Verification items for the finished model (mm, model axes). A direction names the side the tool comes from. Round coordinates to 2 decimals unless told otherwise and drop trailing zeros. Write each loop counter-clockwise with the first axis right and the second up, starting at its lowest first coordinate (ties: lowest second). Pieces come first, ordered by that corner, then holes. Notation, with made-up numbers: M -22.75,49.5 L -0.75,49.5 A16 ccw -0.75,75.5 Z; hole C 54.5,-25 d8. An arc over 180 degrees is marked long. One line per item, written item: value. Start each with the question number.
Item 1: Section check D-D, the plane y = 36. Record the cut outline in (x, z).
Item 2: Thickness scan on probe 1 along X at (y, z) = (-29, 0) (3 decimals); probe 2 along X at (y, z) = (-10.5, 0); probe 3 along X at (y, z) = (26, 0). Record the ranges inside material, lowest first. Write a range as from..to.
Item 3: Gauge pin test, flat ends, axial feed: pin 1 (6 mm diameter, centred on x = 32.5, z = -32, fed in from -Y); pin 2 (6 mm diameter, centred on y = 33.5, z = -19, fed in from -X); pin 3 (3 mm diameter, centred on x = -40, y = -30, fed in from +Z); pin 4 (8 mm diameter, centred on x = 10.5, y = 30.5, fed in from +Z). Record the tip position at first contact, or that the pin passes through.
Item 4: Section check A-A, the plane y = -16.5. Record the cut outline in (x, z) (3 decimals), then the cut area to 3 significant figures.
Item 5: Draft check along X on faces 1 (the face through (18, -30.48, 17)), 2 (the face through (-10.4, 15.24, 10.4)), 3 (the face through (46.492, -23.97, -10.324)). Enter one of: +X half, -X half, draft (parallel to the pull), parting line (faces both ways), or undercut.
Item 6: Tool access check on faces 4 (the face through (-30.911, -6.261, -40.313)), 5 (the face through (0, 20.574, 0)), 6 (the face through (0, 5.08, 0)). Record the directions out of +Z, -Z, +X, -X, +Y, -Y that give a thin tool (end or side, any length) a straight path to the whole face; none if there is none.
from build123d import *

# Parameters (mm, degrees)
SKETCH1_R                = 50.8
SKETCH1_R_2              = 39.116
BOSS_EXTRUDE1_DEPTH      = 12.7
BOSS_EXTRUDE2_DEPTH      = 20.32
BOSS_EXTRUDE2_DEPTH_BACK = 2.54
SKETCH2_R                = 47.625
SKETCH2_R_2              = 39.116
BOSS_EXTRUDE3_DEPTH      = 7.62
BOSS_EXTRUDE3_DEPTH_BACK = 5.08
SKETCH4_R                = 41.91
BOSS_EXTRUDE4_START      = -2.54
SKETCH5_R                = 24.13
BOSS_EXTRUDE4_DEPTH      = 45.72
BOSS_EXTRUDE5_START      = -2.54
SKETCH6_R                = 14.224
BOSS_EXTRUDE5_DEPTH      = 29.21
SKETCH7_R                = 16.51
CUT_EXTRUDE1_DEPTH       = 50.8
SKETCH8_R                = 5.08
CUT_EXTRUDE2_DEPTH       = 26.416


with BuildPart() as part:
    # Sketch1 → Boss-Extrude1 (new body)
    with BuildSketch(Plane(origin=(0, 0, 0), x_dir=(1, 0, 0), z_dir=(0, 1, 0))):
        with Locations(Location((0, 0, 0), (0, 0, 270))):
            Circle(SKETCH1_R)
        with Locations(Location((0, 0, 0), (0, 0, 270))):
            Circle(SKETCH1_R_2, mode=Mode.SUBTRACT)
    extrude(amount=-BOSS_EXTRUDE1_DEPTH)



with BuildPart() as body_2:
    # Sketch2 → Boss-Extrude2 (new, two sides: drawn at the far end of the back side and taken through both)
    with BuildSketch(Plane(origin=(0, -15.24, 0), x_dir=(-1, 0, 0), z_dir=(0, -1, 0)).offset(-BOSS_EXTRUDE2_DEPTH_BACK)):
        with Locations(Location((0, 0, 0), (0, 0, 270))):
            Circle(SKETCH2_R)
        with Locations(Location((0, 0, 0), (0, 0, 270))):
            Circle(SKETCH2_R_2, mode=Mode.SUBTRACT)
    extrude(amount=BOSS_EXTRUDE2_DEPTH + BOSS_EXTRUDE2_DEPTH_BACK)

    # Sketch4 → Boss-Extrude3 (add, two sides: drawn at the far end of the back side and taken through both)
    with BuildSketch(Plane(origin=(0, -38.1, 0), x_dir=(1, 0, 0), z_dir=(0, 1, 0)).offset(-BOSS_EXTRUDE3_DEPTH_BACK)):
        with Locations(Location((0, 0, 0), (0, 0, 270))):
            Circle(SKETCH4_R)
    extrude(amount=BOSS_EXTRUDE3_DEPTH + BOSS_EXTRUDE3_DEPTH_BACK)


with BuildPart() as part_1:
    add(part.part)

    add(body_2.part)  # Boss-Extrude4 merges body 2
    # Sketch5 → Boss-Extrude4 (add)
    with BuildSketch(Plane(origin=(0, -27.94, 0), x_dir=(1, 0, 0), z_dir=(0, 1, 0)).offset(BOSS_EXTRUDE4_START)):
        with Locations(Location((0, 0, 0), (0, 0, 270))):
            Circle(SKETCH5_R)
    extrude(amount=BOSS_EXTRUDE4_DEPTH)

    # Sketch6 → Boss-Extrude5 (add)
    with BuildSketch(Plane(origin=(0, 17.78, 0), x_dir=(1, 0, 0), z_dir=(0, 1, 0)).offset(BOSS_EXTRUDE5_START)):
        with Locations(Location((0, 0, 0), (0, 0, 90))):
            Circle(SKETCH6_R)
    extrude(amount=BOSS_EXTRUDE5_DEPTH)

    # Sketch7 → Cut-Extrude1 (cut)
    with BuildSketch(Plane(origin=(0, -45.72, 0), x_dir=(-1, 0, 0), z_dir=(0, -1, 0))):
        with Locations(Location((0, 0, 0), (0, 0, 90))):
            Circle(SKETCH7_R)
    extrude(amount=-CUT_EXTRUDE1_DEPTH, mode=Mode.SUBTRACT)

    # Sketch8 → Cut-Extrude2 (cut)
    with BuildSketch(Plane(origin=(0, 46.99, 0), x_dir=(1, 0, 0), z_dir=(0, 1, 0))):
        with Locations(Location((0, 0, 0), (0, 0, 270))):
            Circle(SKETCH8_R)
    extrude(amount=-CUT_EXTRUDE2_DEPTH, mode=Mode.SUBTRACT)


solid = part_1.part
Response values:
1. outline: C 0,0 d28.45; hole C 0,0 d10.16
2. probe 1: x = -47.625..-39.116, -24.13..-16.51, 16.51..24.13, 39.116..47.625
2. probe 2: x = -50.8..-39.12, -24.13..-16.51, 16.51..24.13, 39.12..50.8
2. probe 3: x = -14.22..-5.08, 5.08..14.22
3. pin 1: stops at y = -35.56
3. pin 2: passes through
3. pin 3: stops at z = 28.03
3. pin 4: stops at z = 12.65
4. outline: C 0,0 d95.25; C 0,0 d48.26; hole C 0,0 d78.232; hole C 0,0 d33.02
4. area: 3,290 mm2
5. face 1: undercut
5. face 2: draft
5. face 3: parting line
6. face 4: +Y, -Y
6. face 5: +Y
6. face 6: -Y
